The drawing under review shows one solid part. Ordinate dimensions are in mm from its lowest x, y, z. Give positions to 0.01 mm unless a question says otherwise; leave off trailing zeros. Order: outer loops, then holes, each group sorted by start corner. A loop starts at its lowest first (then second) coordinate and runs counter-clockwise, first axis right, second up. Notation, with made-up numbers: (47, 67) -> (64, 67) arc R23 cw to (64, 103) -> close; hole circle Ø3 at (25.5, -28.75). An arc over 180 degrees is marked (long way). One line per item, written item: value. Start each with the question number.
1) The part is to be moulded in two halves that separate along X. For the marked faces 1, 2, 3 and 4, say which applies: released by +X, released by -X, zero draft, split by the parting line, or undercut.
2) Consider section D-D (y = 5). State the section outline as (x, z) points, plus the area to 3 significant figures.
3) Consider section C-C (y = 14.5). State the section outline as (x, z) points, plus the area to 3 significant figures.
4) Wall thickness on line 1 along X through (y, z) = (7, 57); line 2 along X through (y, z) = (20, 57); line 3 along Z through (x, y) = (54.5, 19) (1 decimal): over which ranges is each line inside the solid? List them lowest first. Write a range as from..to.
5) For pin 1 (6 mm diameter, centred on y = 17.5, z = 49.5, fed in from +X); pin 2 (1.5 mm diameter, centred on x = 40, y = 6, fed in from -Z); pin 3 (2 mm diameter, centred on y = 16.5, z = 28.5, fed in from -X), all flat-tipped, find the tip position at first contact; note any pin that passes through.
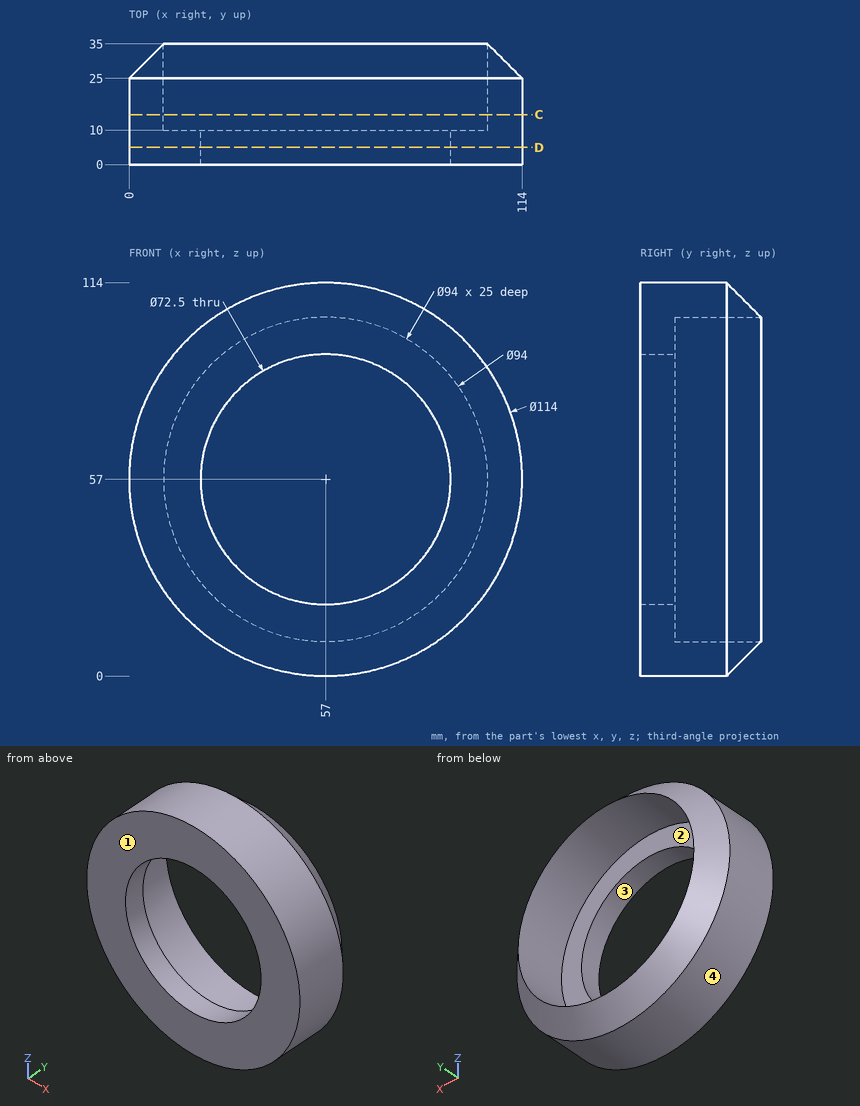
Checked values:
1. face 1: zero draft
1. face 2: undercut
1. face 3: undercut
1. face 4: split by the parting line
2. outline: circle Ø114 at (57, 57); hole circle Ø72.5 at (57, 57)
2. area: 6,080 mm^2
3. outline: circle Ø114 at (57, 57); hole circle Ø94 at (57, 57)
3. area: 3,270 mm^2
4. line 1: x = 0..20.75, 93.25..114
4. line 2: x = 0..10, 104..114
4. line 3: z = 0.1..10.1, 103.9..113.9
5. pin 1: stops at x = 113.82
5. pin 2: stops at z = 2.37
5. pin 3: stops at x = 7.07
